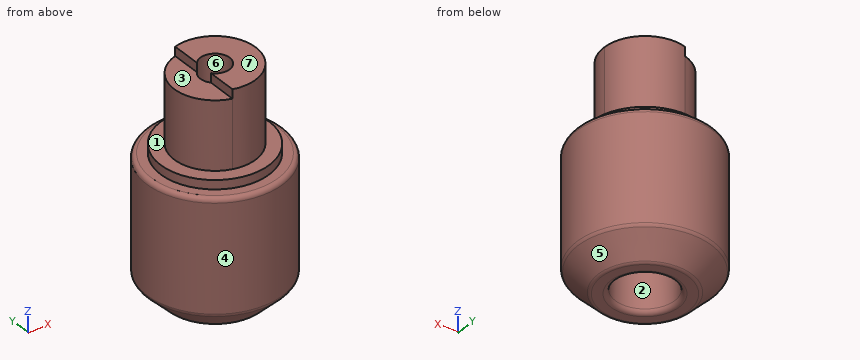
```python
from build123d import *

# Parameters (mm, degrees)
F0_R           = 15
F1_DEPTH       = 30
F2_R           = 12
F3_DEPTH       = 2
F5_DEPTH       = 17
F6_DEPTH       = 15
F7_D           = 6.5
F7_CBORE_D     = 13
F7_CBORE_DEPTH = 15
F8_SIZE        = 5
F9_R           = 1


with BuildPart() as f1:
    # F0 (on Top) → F1 (new body)
    with BuildSketch(Plane.XY):
        Circle(F0_R)
    extrude(amount=F1_DEPTH)

    # F2 (on face) → F3 (join)
    with BuildSketch(Plane.XY.offset(30)):
        Circle(F2_R)
    extrude(amount=F3_DEPTH)

    # F4 (on face) → F5 (join)
    with BuildSketch(Plane.XY.offset(32)):
        with BuildLine():
            ThreePointArc((-2.4664324925, -8.6554439955), (5.4222738573, -7.1832406486), (9, 0))
            ThreePointArc((9, 0), (5.4222738573, 7.1832406486), (-2.4664324925, 8.6554439955))
            Line((-2.4664324925, 8.6554439955), (-2.4664324925, -8.6554439955))
        make_face()
    extrude(amount=F5_DEPTH)

    # F4 (on face) → F6 (join)
    with BuildSketch(Plane.XY.offset(32)):
        with BuildLine():
            Line((-2.4664324925, -8.6554439955), (-2.4664324925, 8.6554439955))
            ThreePointArc((-2.4664324925, 8.6554439955), (-9, 0), (-2.4664324925, -8.6554439955))
        make_face()
    extrude(amount=F6_DEPTH)

    # F7 (through all)
    with Locations(Plane(origin=(0, 0, 0), x_dir=(1, 0, 0), z_dir=(0, 0, -1))):
        with Locations((0, 0)):
            CounterBoreHole(F7_D / 2, F7_CBORE_D / 2, F7_CBORE_DEPTH)

    # F8
    f8_edges = [f1.edges().sort_by_distance(p)[0] for p in [
        (-15, 0, 0),
    ]]
    chamfer(f8_edges, length=F8_SIZE)

    # F9
    f9_edges = [f1.edges().sort_by_distance(p)[0] for p in [
        (-15, 0, 30),
        (-10, 0, 0),
        (-15, 0, 5),
        (-6.5, 0, 0),
    ]]
    fillet(f9_edges, radius=F9_R)


solid = f1.part
```
Work out the finished part from the listing and answer in its coordinate system (mm). Face numbers are marked on the shaded views. A direction names the side the tool comes from. Give positions to 0.01 mm unless a question says otherwise; leave off trailing zeros. Order: outer loops, then holes, each group sorted by start corner. A loop starts at its lowest first (then second) coordinate and runs counter-clockwise, first axis right, second up.
1. Straight lines are drawn through the part: L1, parallel to Y at x = 0, z = 7; L2, parallel to Y at x = 0, z = 37. For each, find the intervals that lie inside material, in ascending order.
Result sheet:
L1: y = -15 to -6.5, 6.5 to 15
L2: y = -9 to -3.25, 3.25 to 9
2. Section A-A, the plane z = 39 is taken. Determine the outline of the cut face in (x, y), and give its area (3 significant figures).
Result sheet:
outline: circle Ø18 at (0, 0); hole circle Ø6.5 at (0, 0)
area: 221 mm2
3. For the marked faces 1, 2, 3 and 4, determine the directions among +Z, -Z, +X, -X, +Y, -Y from which every point of the face is accessible in a straight line to the end or side of a thin tool.
Result sheet:
face 1: +Z
face 2: -Z
face 3: +Z, -X, +Y, -Y
face 4: +Z, -Z
4. Each of these flat-tipped pins is pushed along its axis until it touches: P1, Ø1.5, axis at y = 3, z = 35.5, coming from the -X side; P2, Ø1.5, axis at x = 9, z = 25, coming from the +Y side; P3, Ø4, axis at x = -1.5, y = -1, coming from the -Z side. Where does it stop, or does it pass through?
Result sheet:
P1: stops at x = -8.71
P2: stops at y = 12.53
P3: stops at z = 15
5. Section B-B, the plane z = 7.5 is taken. Determine the outline of the cut face in (x, y), and give its area (3 significant figures).
Result sheet:
outline: circle Ø30 at (0, 0); hole circle Ø13 at (0, 0)
area: 574 mm2
6. Section C-C, the plane z = 25.5 is taken. Determine the outline of the cut face in (x, y), and give its area (3 significant figures).
Result sheet:
outline: circle Ø30 at (0, 0); hole circle Ø6.5 at (0, 0)
area: 674 mm2
7. The mould has two halves that part along Y. Classify the marked faces 5, 6 and 7: released by +Y, released by -Y, zero draft, split by the parting line, or undercut.
Result sheet:
face 5: split by the parting line
face 6: undercut
face 7: zero draft
